Source: three-view drawing plus pictorial views. Frame: mm from the lowest corner of the part. Round coordinates to 2 decimals unless told otherwise and drop trailing zeros. Write each loop counter-clockwise with the first axis right and the second up, starting at its lowest first coordinate (ties: lowest second). Pieces come first, ordered by that corner, then holes.
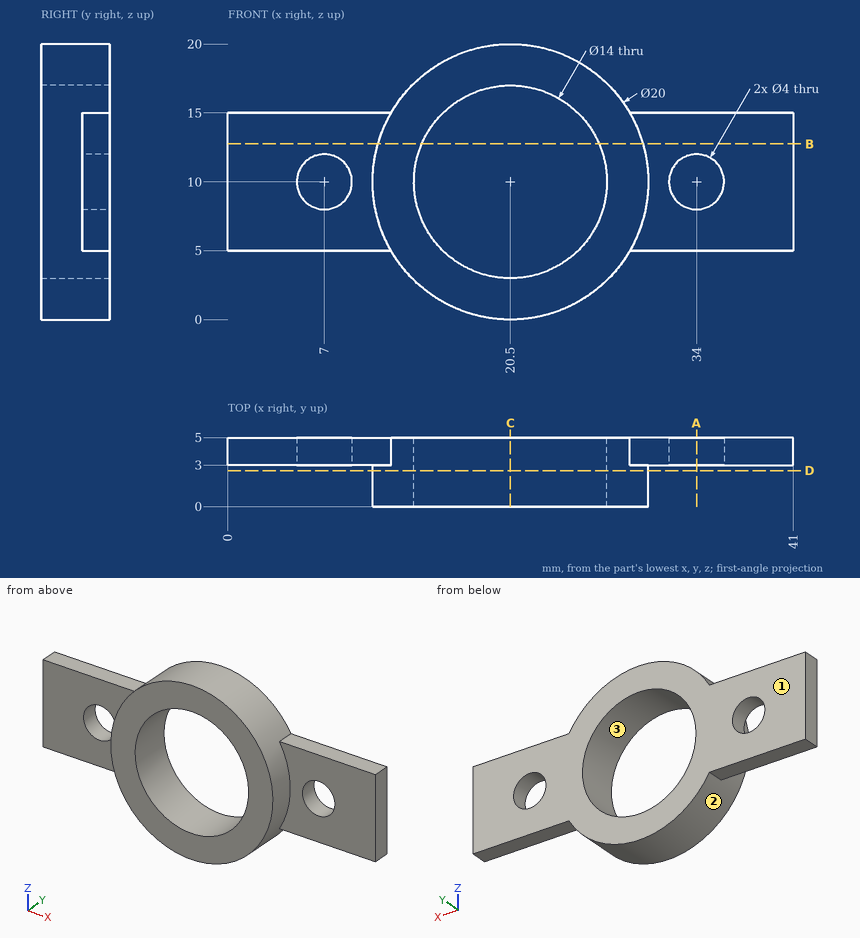
1) Line query: probe 1 along X at (y, z) = (4.3, 10); probe 2 along Y at (x, z) = (8.5, 8.5); probe 3 along X at (y, z) = (4.05, 7). Output: solid intervals per line, ascending.
2) Section A-A on x = 34. Output: boundary loops of the cut face in (y, z).
3) First-contact query: P1, Ø11, axis at x = 4, z = 10.5, coming from the -Y side; P2, Ø1.5, axis at x = 17.5, y = 3, coming from the +Z side; P3, Ø1, axis at x = 34, y = 4.5, coming from the -Z side. Flat tips, straight axial feed; report the tip coordinate or a pass-through.
4) Draft query along Z for the marked faces 1, 2 and 3. Return one class per face: pulls with the +Z half, pulls with the -Z half, needs draft (parallel to the pull), parting line crosses it, or undercut.
5) Section B-B on z = 12.75. Output: boundary loops of the cut face in (x, y).
6) Section C-C on x = 20.5. Output: boundary loops of the cut face in (y, z).
7) Section D-D on y = 2.6. Output: boundary loops of the cut face in (x, z).
Filled in:
1. probe 1: x = 0 to 5, 9 to 13.5, 27.5 to 32, 36 to 41
1. probe 2: y = 3 to 5
1. probe 3: x = 0 to 14.18, 26.82 to 41
2. outline: (3, 5) - (5, 5) - (5, 8) - (3, 8) - close; (3, 12) - (5, 12) - (5, 15) - (3, 15) - close
3. P1: stops at y = 3
3. P2: stops at z = 19.74
3. P3: stops at z = 5
4. face 1: needs draft
4. face 2: parting line crosses it
4. face 3: undercut
5. outline: (0, 3) - (10.89, 3) - (10.89, 0) - (14.06, 0) - (14.06, 5) - (0, 5) - close; (26.94, 0) - (30.11, 0) - (30.11, 3) - (41, 3) - (41, 5) - (26.94, 5) - close
6. outline: (0, 0) - (5, 0) - (5, 3) - (0, 3) - close; (0, 17) - (5, 17) - (5, 20) - (0, 20) - close
7. outline: circle Ø20 at (20.5, 10); hole circle Ø14 at (20.5, 10)
